from build123d import *

# Parameters (mm, degrees)
F0_R      = 135
F1_DEPTH  = 1600
F2_R      = 10
F6_DEPTH  = 5
F5_R      = 10
F7_DEPTH  = 25
F8_T      = -3
F9_R      = 8.5
F10_DEPTH = 50
F11_R     = 10
F11_R_2   = 7.5


with BuildPart() as f1:
    # F0 (on Top) → F1 (new body)
    with BuildSketch(Plane.XY):
        Circle(F0_R)
    extrude(amount=F1_DEPTH)

    # F2 (on face) → F6 (join)
    with BuildSketch(Plane.XY.offset(1600)):
        Circle(F2_R)
    extrude(amount=F6_DEPTH)

    # F5 (on offset) → F7 (join)
    with BuildSketch(Plane.XZ.offset(-125)):
        with Locations((0, 1565)):
            Circle(F5_R)
    extrude(amount=-F7_DEPTH)

    # F8
    f8_openings = [f1.faces().sort_by_distance(p)[0] for p in [
        (0, 0, 0),
    ]]
    offset(amount=F8_T, openings=f8_openings, kind=Kind.INTERSECTION)

    # F9 (on face) → F10 (cut)
    with BuildSketch(Plane(origin=(0, 150, 0), x_dir=(-1, 0, 0), z_dir=(0, 1, 0))):
        with Locations((0, 1565)):
            Circle(F9_R)
    extrude(amount=-F10_DEPTH, mode=Mode.SUBTRACT)

    # F12: sweep along a path in F3
    with BuildLine(Plane.YZ) as f12_path:
        Line((0, 1600), (0, 1620))
        ThreePointArc((0, 1620), (8.7867965644, 1641.2132034356), (30, 1650))
        Line((30, 1650), (200, 1650))
    # F11 (on face) → F12 (sweep)
    with BuildSketch(Plane.XY.offset(1605)):
        Circle(F11_R)
        Circle(F11_R_2, mode=Mode.SUBTRACT)
    sweep(path=f12_path.line)


solid = f1.part
Here's how the part is built. I have some questions about the finished solid (model axes, mm). A direction names the side the tool comes from. Round coordinates to 2 decimals unless told otherwise and drop trailing zeros. Order: outer loops, then holes, each group sorted by start corner. A loop starts at its lowest first (then second) coordinate and runs counter-clockwise, first axis right, second up. Notation, with made-up numbers: (10, 86.5) -> (54, 86.5) arc R25 ccw to (54, 111.5) -> close; hole circle Ø2 at (66, 87.5). An arc over 180 degrees is marked (long way). Use CSV: the item, a comma, the result in double quotes.
1. I want a section at A-A on y = 50.5. List the corners of the cut face in (x, z) for me.
Recorded:
outline,"(-125.2, 0) -> (-121.96, 0) -> (-121.96, 1597) -> (121.96, 1597) -> (121.96, 0) -> (125.2, 0) -> (125.2, 1600) -> (-125.2, 1600) -> close; circle Ø20 at (0, 1650); hole circle Ø15 at (0, 1650)"
2. I need wall thicknesses on line 1 along X through (y, z) = (146, 1565); line 2 along Z through (x, y) = (0, 111.5); line 3 along Z through (x, y) = (-2, 102.5). Which ranges of each line are inside material? Lowest first, please.
Recorded:
line 1,"x = -10 to -8.5, 8.5 to 10"
line 2,"z = 1597 to 1600, 1640 to 1642.5, 1657.5 to 1660"
line 3,"z = 1597 to 1600, 1640.2 to 1642.77, 1657.23 to 1659.8"
3. I want a section at B-B on x = 71. List the corners of the cut face in (y, z) for me.
Recorded:
outline,"(-114.82, 0) -> (-111.28, 0) -> (-111.28, 1597) -> (111.28, 1597) -> (111.28, 0) -> (114.82, 0) -> (114.82, 1600) -> (-114.82, 1600) -> close"
4. Which directions (+Z, -Z, +X, -X, +Y, -Y) give clear straight access to the entire face, cutting with the end or side of a thin tool? Please do faces 1 (the face through (129, -29, 0)), 2 (the face through (121.934, -50.557, 787.321)).
Recorded:
face 1,"-Z, +X, -X, +Y, -Y"
face 2,"-Z"
5. I'm going to push flat-ended pins straight in: P1, Ø1.5, axis at y = 52.5, z = 727.5, coming from the -X side; P2, Ø5, axis at x = 90.5, y = 59.5, coming from the +Z side; P3, Ø1, axis at x = -6, z = 941.5, coming from the -Y side; P4, Ø17, axis at x = 0, z = 1650, coming from the +Y side. Where does each tip first touch, or does it pass through?
Recorded:
P1,"stops at x = -124.69"
P2,"stops at z = 1600"
P3,"stops at y = -134.89"
P4,"stops at y = 200"
6. I want a section at C-C on z = 1086. List the corners of the cut face in (x, y) for me, and give its area (3 significant figures).
Recorded:
outline,"circle Ø270 at (0, 0); hole circle Ø264 at (0, 0)"
area,"2,520 mm2"
7. I want a section at D-D on x = -86.5. List the corners of the cut face in (y, z) for me, and give its area (3 significant figures).
Recorded:
outline,"(-103.65, 0) -> (-99.71, 0) -> (-99.71, 1597) -> (99.71, 1597) -> (99.71, 0) -> (103.65, 0) -> (103.65, 1600) -> (-103.65, 1600) -> close"
area,"13,200 mm2"
8. Thinking about a two-plate mould opening in Y: for faces 3 (the face through (-107.13, -82.15, 788.8)), 4 (the face through (-2, -27, 1597)), 5 (the face through (-2, -28, 1600)), which applies, pulls with the +Y half, pulls with the -Y half, needs draft (parallel to the pull), parting line crosses it, or undercut?
Recorded:
face 3,"parting line crosses it"
face 4,"undercut"
face 5,"needs draft"
